Could you check a few things on this model? Use its own coordinates, in mm. A direction names the side the tool comes from. Give positions to 0.01 mm unless a question says otherwise; leave off trailing zeros. Write each loop counter-clockwise with the first axis right and the second up, starting at its lowest first coordinate (ties: lowest second). Pieces come first, ordered by that corner, then holes. Notation, with made-up numbers: (48.5, 60.25) - (56.5, 60.25) arc R28 cw to (56.5, 81.25) - close; hole circle Ø3 at (22, -35). An arc over 180 degrees is marked (long way). Answer in a Markdown table with one row per item.
Autodesk Inventor part; units mm, degrees
ref_plane "Work Plane1" through (1.75, 0, 0) normal (0, 0, -1) x (1, 0, 0)
ref_plane "YZ Plane" through (0, 0, 0) normal (1, 0, 0) x (0, 1, 0)
ref_plane "XZ Plane" through (0, 0, 0) normal (0, 1, 0) x (-1, 0, 0)
sketch "Sketch1" plane through (0, 0, 0) normal (0, 0, 1) x (1, 0, 0)
  line L0 (0, 3.175) -> (82.55, 3.175)
  line L1 (82.55, 3.175) -> (82.55, 0)
  line L2 (82.55, 0) -> (0, 0)
  line L3 (0, 0) -> (0, 3.175)
  line L4 (0, -0.635) -> (0, 3.81)
  line L5 (-16.51, 0) -> (99.06, 0)
  dimension "d1" = 6.35
  dimension "d13" = 82.55
revolve "Body" add sketch "Sketch1" angle 360 about axis through (82.55, 0, 0) along (-1, 0, 0)
sketch "Sketch2" plane through (0, 0, 0) normal (-1, 0, 0) x (0, 0, 1)
  line L0 (0, 6.4231) -> (5.5626, 3.2116)
  line L1 (5.5626, 3.2116) -> (5.5626, -3.2116)
  line L2 (5.5626, -3.2116) -> (0, -6.4231)
  line L3 (0, -6.4231) -> (-5.5626, -3.2116)
  line L4 (-5.5626, -3.2116) -> (-5.5626, 3.2116)
  line L5 (-5.5626, 3.2116) -> (0, 6.4231)
  line L6 (-7.7876, 0) -> (7.7876, 0)
  line L7 (0, 8.9924) -> (0, -8.9924)
  point P0 (0, 0)
  point P1 (0, 0)
  point P2 (0, 0)
  dimension "d8" = 11.1252
extrude "Head" add sketch "Sketch2" along normal blind 4.826
sketch "Sketch3" plane through (-4.826, 0, 0) normal (-1, 0, 0) x (0, 0, 1)
  circle A0 centre (0, 0) radius 4.4501
  point P0 (0, 0)
  dimension "d18" = 8.9002
extrude "Indent" cut sketch "Sketch3" against normal blind 0.4836
sketch "Sketch4" plane through (0, 0, 0) normal (0, 0, 1) x (1, 0, 0)
  line L0 (-4.826, 5.5626) -> (-4.826, 6.4231)
  line L1 (-4.826, 6.4231) -> (-4.3292, 6.4231)
  line L2 (-4.3292, 6.4231) -> (-4.826, 5.5626)
  line L3 (-5.7912, 0) -> (0.9652, 0)
  line L4 (0, 6.4231) -> (-4.826, 6.4231)
  line L5 (-4.826, 3.2116) -> (-4.826, 6.4231)
  dimension "d4" = 30
  dimension "d17" = 11.1252
revolve "Chamfer1" cut sketch "Sketch4" angle 360 about axis through (-10, 0, 0) along (1, 0, 0)
thread "Thread"
chamfer "Chamfer2" distance 0.635 distance2 0.6351 1 edges at (82.55, -3.175, 0) measured on face at (82.55, 0.6012, 0.871)
ref_plane "Work Plane1" through (1.75, 0, 0) normal (0, 0, -1) x (1, 0, 0)
equation "\"d1\" = GD"
equation "\"d13\" = NLG"
equation "\"d8\" = SW"
equation "\"d2\" = KOH - SD"
equation "\"d18\" = KOD2"
equation "\"d4\" = ANG1"
equation "\"d17\" = SW"
equation "\"d9\" = GEL"
equation "\"d5\" = -0.5 * SPD + 0.5 * GD"
equation "\"NLG\" = 82.55"
equation "\"GD\" = NND"
equation "\"BDM\" = NND"
equation "\"KOH\" = 4.826"
equation "\"GEL\" = 70.1675"
equation "\"SW\" = 11.1252"
equation "\"SPD\" = GD1"
equation "\"SD\" = 0"
equation "\"ANG1\" = 30deg"
equation "\"GAL\" = 0.635"
equation "\"GUL\" = GAL"
equation "\"KOH2\" = 0.1 * KOH"
equation "\"KOD2\" = 0.8 * SW"
equation "\"GD1\" = 5.08"
equation "\"THREADDIA\" = 6.35"
equation "\"SDH\" = SW"
equation "\"TOA\" = 30deg"
equation "\"RR\" = 0.0635"
equation "\"NND\" = 6.35"
equation "\"SW0\" = SW"
equation "\"SD2\" = NND"
equation "\"E0\" = 1.155 * SW"
properties part number "ANSI B18.6.3 - 1/4-20 UNC - 3.25" material "Steel, Mild"
1) Imagine slicing it at A-A (x = 15.5). List the corners of the cut face in (y, z) for me (3 decimals).
Check values:
| item | result |
|---|---|
| outline | circle Ø6.35 at (0, 0) |
2) Will these pins go through, and if not, where does the flat tip stop? P1, Ø4.5, axis at y = 1, z = -1, coming from the -X side; P2, Ø5, axis at x = 45, z = -4, coming from the +Y side; P3, Ø6, axis at x = 67.5, z = 1.5, coming from the +Y side (3 decimals).
Check values:
| item | result |
|---|---|
| P1 | stops at x = -4.34 |
| P2 | stops at y = 2.8 |
| P3 | stops at y = 3.175 |
3) If I drill on line 1 (X direction, y = 0.75, z = 0); line 2 (Y direction, x = -4.5, z = 0); line 3 (Y direction, x = 52.5, z = -1.5), over which ranges is the centre line in solid material (lowest first)?
Check values:
| item | result |
|---|---|
| line 1 | x = -4.34 to 82.55 |
| line 2 | y = -6.13 to -4.45, 4.45 to 6.13 |
| line 3 | y = -2.8 to 2.8 |
4) On a 3-axis mill with a long thin cutter (end or side, diameter ignored), from which of +Z, -Z, +X, -X, +Y, -Y can I reach the whole of each face in a straight line? I mean faces 5 (the face through (-4.7, -2.9, -5)), 6 (the face through (41.53, -0.69, -3.1)). Say none if no direction works.
Check values:
| item | result |
|---|---|
| face 5 | -Z, -X, -Y |
| face 6 | +X |
5) We'd pull the mould along Y, two halves only. Please class faces 1 (the face through (-2, 0, -5.563)), 2 (the face through (-4.705, 5.772, -0.014)), 3 (the face through (-4.342, 0, 0)), 4 (the face through (-4.588, 4.412, -0.579)): +Y half, -Y half, draft (parallel to the pull), parting line (faces both ways), or undercut.
Check values:
| item | result |
|---|---|
| face 1 | draft |
| face 2 | +Y half |
| face 3 | undercut |
| face 4 | undercut |
